from build123d import *

# Parameters (mm, degrees)
SKETCH1_W           = 100
SKETCH1_H           = 50
SKETCH1_R           = 10
SKETCH1_R_2         = 2.5
BOSS_EXTRUDE1_DEPTH = 5
SKETCH2_R           = 4.5
CUT_EXTRUDE1_DEPTH  = 3


with BuildPart() as part:
    # Sketch1 → Boss-Extrude1 (new body)
    with BuildSketch(Plane(origin=(0, 0, 0), x_dir=(1, 0, 0), z_dir=(0, 1, 0))):
        Rectangle(SKETCH1_W, SKETCH1_H)
        with Locations(Location((30, 0, 0), (0, 0, 270))):
            Circle(SKETCH1_R, mode=Mode.SUBTRACT)
        with Locations(Location((-30, 0, 0), (0, 0, 270))):
            Circle(SKETCH1_R, mode=Mode.SUBTRACT)
        with Locations(Location((44, 19, 0), (0, 0, 270))):
            Circle(SKETCH1_R_2, mode=Mode.SUBTRACT)
        with Locations(Location((-44, 19, 0), (0, 0, 270))):
            Circle(SKETCH1_R_2, mode=Mode.SUBTRACT)
        with Locations(Location((-44, -19, 0), (0, 0, 270))):
            Circle(SKETCH1_R_2, mode=Mode.SUBTRACT)
        with Locations(Location((44, -19, 0), (0, 0, 270))):
            Circle(SKETCH1_R_2, mode=Mode.SUBTRACT)
    extrude(amount=BOSS_EXTRUDE1_DEPTH)

    # Sketch2 → Cut-Extrude1 (cut)
    with BuildSketch(Plane(origin=(0, 5, 0), x_dir=(1, 0, 0), z_dir=(0, 1, 0))):
        with Locations(Location((-44, 19, 0), (0, 0, 270))):
            Circle(SKETCH2_R)
        with Locations(Location((-44, -19, 0), (0, 0, 270))):
            Circle(SKETCH2_R)
        with Locations(Location((44, -19, 0), (0, 0, 270))):
            Circle(SKETCH2_R)
        with Locations(Location((44, 19, 0), (0, 0, 270))):
            Circle(SKETCH2_R)
    extrude(amount=-CUT_EXTRUDE1_DEPTH, mode=Mode.SUBTRACT)


solid = part.part
The listing builds one solid part. Answer for the finished solid, in the listing's coordinates (mm). A direction names the side the tool comes from. Round coordinates to 2 decimals unless told otherwise and drop trailing zeros. Order: outer loops, then holes, each group sorted by start corner. A loop starts at its lowest first (then second) coordinate and runs counter-clockwise, first axis right, second up. Notation, with made-up numbers: (12, -13.75) -> (66, -13.75) arc R12 cw to (66, 3.25) -> close; hole circle Ø4 at (66, 41.5). An arc over 180 degrees is marked (long way). One line per item, written item: value.
Item 1: Find section B-B, the plane x = 44. Give the vertices of the cut face in (y, z).
Taken from the geometry:
outline: (0, -25) -> (5, -25) -> (5, -23.5) -> (2, -23.5) -> (2, -21.5) -> (0, -21.5) -> close; (0, -16.5) -> (2, -16.5) -> (2, -14.5) -> (5, -14.5) -> (5, 14.5) -> (2, 14.5) -> (2, 16.5) -> (0, 16.5) -> close; (0, 21.5) -> (2, 21.5) -> (2, 23.5) -> (5, 23.5) -> (5, 25) -> (0, 25) -> close
Item 2: For faces 4 (the flat face through (-1, 0, 0)), 5 (the cylindrical face through (39.61, 3.52, 18.02)), determine the directions among +Z, -Z, +X, -X, +Y, -Y from which every point of the face is accessible in a straight line to the end or side of a thin tool.
Taken from the geometry:
face 4: +Z, -Z, +X, -X, -Y
face 5: +Y
Item 3: For a pull along Z with two mould halves and no side action, classify faces 1 (the flat face through (50, 2, 0)), 2 (the flat face through (-1, 2, 25)), 3 (the cylindrical face through (-45.5, 1, 17)) as released by +Z, released by -Z, zero draft, split by the parting line, or undercut.
Taken from the geometry:
face 1: zero draft
face 2: released by +Z
face 3: undercut
Item 4: Find section A-A, the plane z = 19. Give the vertices of the cut face in (x, y), then the cut area to 3 significant figures.
Taken from the geometry:
outline: (-50, 0) -> (-46.5, 0) -> (-46.5, 2) -> (-48.5, 2) -> (-48.5, 5) -> (-50, 5) -> close; (-41.5, 0) -> (41.5, 0) -> (41.5, 2) -> (39.5, 2) -> (39.5, 5) -> (-39.5, 5) -> (-39.5, 2) -> (-41.5, 2) -> close; (46.5, 0) -> (50, 0) -> (50, 5) -> (48.5, 5) -> (48.5, 2) -> (46.5, 2) -> close
area: 426 mm2
Item 5: Straight lines are drawn through the part: L1, parallel to X at y = 0.7, z = 19; L2, parallel to Z at x = 44, y = 0.4; L3, parallel to X at y = 1.2, z = -5.5. For each, find the intervals that lie inside material, in ascending order.
Taken from the geometry:
L1: x = -50 to -46.5, -41.5 to 41.5, 46.5 to 50
L2: z = -25 to -21.5, -16.5 to 16.5, 21.5 to 25
L3: x = -50 to -38.35, -21.65 to 21.65, 38.35 to 50
Item 6: Given P1, Ø2.5, axis at x = 45.5, z = -21, coming from the +Y side, flat-ended and moving along its own axis, determine where the tip first touches the part or whether it passes through.
Taken from the geometry:
P1: stops at y = 2
Item 7: Find section D-D, the plane y = 3.35. Give the vertices of the cut face in (x, z).
Taken from the geometry:
outline: (-50, -25) -> (50, -25) -> (50, 25) -> (-50, 25) -> close; hole circle Ø9 at (-44, -19); hole circle Ø9 at (-44, 19); hole circle Ø20 at (-30, 0); hole circle Ø20 at (30, 0); hole circle Ø9 at (44, -19); hole circle Ø9 at (44, 19)
Item 8: Find section C-C, the plane x = -30. Give the vertices of the cut face in (y, z), then the cut area to 3 significant figures.
Taken from the geometry:
outline: (0, -25) -> (5, -25) -> (5, -10) -> (0, -10) -> close; (0, 10) -> (5, 10) -> (5, 25) -> (0, 25) -> close
area: 150 mm2
